from build123d import *

# Parameters (mm, degrees)
F1_DEPTH      = 68.834
F3_DEPTH      = 56.642
F4_DEPTH      = 21.59
F6_DEPTH      = 16.256
F7_T1_DEPTH   = 134.6089194051
F8_SIZE       = 5.08
F9_T4_DEPTH   = 246.1695934192
F9_T9_DEPTH   = 246.1695934192
F11_DEPTH     = 13.97
F12_T1_DEPTH  = 239.1129526059
F12_T6_DEPTH  = 239.1129526059
F13_W         = 8.2417714845
F13_H         = 1.1003240943
F14_DEPTH     = 1.524
F16_DEPTH     = 13.208
F17_T1_DEPTH  = 236.9807138407
F17_T6_DEPTH  = 236.9807138407
F17_T12_DEPTH = 236.9807138407
F17_T18_DEPTH = 236.9807138407


# Not quite as in the source:
# - a fillet or chamfer that OpenCascade refuses, or shapes differently, is made with other operations: its cross-section is extruded or revolved along the edge and cut away or added


with BuildPart() as f1:
    # F0 (on Front) → F1 (new body)
    with BuildSketch(Plane.XZ):
        with BuildLine():
            Line((-134.6334815025, -70.4434812069), (236.5282326937, -70.4434812069))
            Line((236.5282326937, -70.4434812069), (201.5823870897, -52.4187758565))
            add(Edge.make_bspline(
                [(201.5823870897, -52.4187758565), (186.6945113423, -52.7201094998), (157.86128429, -53.3036998994), (136.5029788289, -38.0790520799), (126.1729151011, -30.7155661285)],
                knots=[0, 0, 0, 0, 0.5163444147, 1, 1, 1, 1], degree=3))
            Line((126.1729151011, -30.7155661285), (57.3847740889, -6.4373956993))
            Line((57.3847740889, -6.4373956993), (-104.8375442624, -52.4187758565))
            Line((-104.8375442624, -52.4187758565), (-134.6334815025, -70.4434812069))
        make_face()
    extrude(amount=-F1_DEPTH)

    # F2 (on face) → F3 (join)
    with BuildSketch(Plane(origin=(0, 68.834, 0), x_dir=(-1, 0, 0), z_dir=(0, 1, 0))):
        Polygon((104.8375442624, -52.4187758565), (-57.3847740889, -6.4373956993), (-57.3847740889, -70.4434812069), (134.6334815025, -70.4434812069), align=None)
    extrude(amount=F3_DEPTH)

    # F4 (add): a face of the model
    f4_faces = [f1.faces().sort_by_distance(p)[0] for p in [
        (117.597457412, 68.834, -49.4942566091),
    ]]
    extrude(f4_faces, amount=F4_DEPTH)

    # F5 (on face) → F6 (join)
    with BuildSketch(Plane(origin=(0, 90.424, 0), x_dir=(-1, 0, 0), z_dir=(0, 1, 0))):
        Polygon((-284.8027348518, -56.1655424535), (-284.8027348518, -70.4434812069), (-57.3847740889, -70.4434812069), (-57.3847740889, 0), align=None)
    extrude(amount=F6_DEPTH)

    # F7: chamfer of 22.86 x 14.478 on 1 edges, made by hand

    # F7_s2 → F7_t1 (cut)
    with BuildSketch(Plane.XZ.offset(-165.8564597025)):
        Polygon((262.6095480908, -50.6844785612), (284.8027348518, -70.6435424535), (284.8027348518, -56.1655424535), align=None)
    extrude(amount=F7_T1_DEPTH, mode=Mode.SUBTRACT)

    # F8
    f8_edges = [f1.edges().sort_by_distance(p)[0] for p in [
        (57.384774, 98.552, 0),
    ]]
    chamfer(f8_edges, length=F8_SIZE)

    # F9: fillet of radius 7.971733183 on 2 edges, made by hand


with BuildPart() as f9_tool2:
    # F9_s3 → F9_t4 (new body)
    with BuildSketch(Plane(origin=(39.6696512747, 0, -9.7972362223), x_dir=(0, 1, 0), z_dir=(0.970830567, 0, -0.2397665745))):
        with BuildLine():
            ThreePointArc((106.68, 5.7872175269), (104.3451334085, 11.4240841184), (98.708266817, 13.7589507099))
            Line((98.708266817, 13.7589507099), (106.68, 13.7589507099))
            Line((106.68, 13.7589507099), (106.68, 5.7872175269))
        make_face()
    extrude(amount=F9_T4_DEPTH)

    split(bisect_by=Plane.YZ.offset(57.3847740889), keep=Keep.TOP)


with BuildPart() as f1_1:
    add(f1.part)

    # F9_t1: cut F9_tool2
    add(f9_tool2.part, mode=Mode.SUBTRACT)


with BuildPart() as f9_tool7:
    # F9_s8 → F9_t9 (new body)
    with BuildSketch(Plane(origin=(39.6696512747, 0, -9.7972362223), x_dir=(0, 1, 0), z_dir=(0.970830567, 0, -0.2397665745))):
        with BuildLine():
            ThreePointArc((90.424, 5.7872175269), (92.7588665915, 11.4240841184), (98.395733183, 13.7589507099))
            Line((98.395733183, 13.7589507099), (90.424, 13.7589507099))
            Line((90.424, 13.7589507099), (90.424, 5.7872175269))
        make_face()
    extrude(amount=F9_T9_DEPTH)

    split(bisect_by=Plane(origin=(4.3361166105, 0, 12.285662205), x_dir=(0, 1, 0), z_dir=(0.3328201545, 0, 0.9429903206)), keep=Keep.TOP)


with BuildPart() as f1_2:
    add(f1_1.part)

    # F9_t6: cut F9_tool7
    add(f9_tool7.part, mode=Mode.SUBTRACT)

    # F10 (on face) → F11 (join)
    with BuildSketch(Plane(origin=(0, 125.476, 0), x_dir=(-1, 0, 0), z_dir=(0, 1, 0))):
        Polygon((-45.8267219365, -2.2306151222), (-57.3847740889, -6.4373956993), (104.8375442624, -52.4187758565), (134.6334815025, -70.4434812069), (161.1742377281, -70.4434812069), (150.1698791981, -52.4187758565), align=None)
    extrude(amount=-F11_DEPTH)

    # F12: fillet of radius 7.3585229381 on 2 edges, made by hand

    # F12_s2 → F12_t1 (cut)
    with BuildSketch(Plane(origin=(-171.3471837913, 0, -43.8762710766), x_dir=(0, 1, 0), z_dir=(0.9687439392, 0, 0.2480628554))):
        with BuildLine():
            ThreePointArc((118.1174770619, -13.5288023788), (123.3207385309, -15.6840638479), (125.476, -20.8873253169))
            Line((125.476, -20.8873253169), (125.476, -13.5288023788))
            Line((125.476, -13.5288023788), (118.1174770619, -13.5288023788))
        make_face()
    extrude(amount=F12_T1_DEPTH, mode=Mode.SUBTRACT)


with BuildPart() as f12_tool4:
    # F12_s5 → F12_t6 (new body)
    with BuildSketch(Plane(origin=(-171.3471837913, 0, -43.8762710766), x_dir=(0, 1, 0), z_dir=(0.9687439392, 0, 0.2480628554))):
        with BuildLine():
            ThreePointArc((118.8645229381, -13.5288023788), (113.6612614691, -15.6840638479), (111.506, -20.8873253169))
            Line((111.506, -20.8873253169), (111.506, -13.5288023788))
            Line((111.506, -13.5288023788), (118.8645229381, -13.5288023788))
        make_face()
    extrude(amount=F12_T6_DEPTH)

    split(bisect_by=Plane(origin=(5.9565096776, 0, -21.0145673287), x_dir=(0, 1, 0), z_dir=(-0.272703532, 0, 0.9620981154)), keep=Keep.TOP)


with BuildPart() as f1_3:
    add(f1_2.part)

    # F12_t3: cut F12_tool4
    add(f12_tool4.part, mode=Mode.SUBTRACT)

    # F13 (on face) → F14 (join)
    with BuildSketch(Plane(origin=(5.9565096776, 0, -21.0145673287), x_dir=(0.9620981154, 0, 0.272703532), z_dir=(-0.272703532, 0, 0.9620981154))):
        with Locations((49.3333967155, 86.9543515146)):
            Rectangle(F13_W, F13_H)
    extrude(amount=F14_DEPTH)

    # F15 (on face) → F16 (join)
    with BuildSketch(Plane.XZ.offset(-86.4041894674)):
        Polygon((-104.8238277435, -52.4797327816), (57.3847740889, -6.4373956993), (46.4603118598, -2.0644166507), (-150.4420638084, -52.4797327816), (-161.1757725477, -70.3692361712), (-134.1178864241, -70.3692361712), align=None)
    extrude(amount=F16_DEPTH)

    # F17: fillet of radius 6.7453126933 on 2 edges, made by hand

    # F17_s2 → F17_t1 (cut)
    with BuildSketch(Plane(origin=(59.4421171299, 0, 15.219690044), x_dir=(0, 1, 0), z_dir=(-0.9687495941, 0, -0.2480407708))):
        with BuildLine():
            ThreePointArc((73.1961894674, 20.2692670518), (75.1718458141, 15.4996107052), (79.9415021607, 13.5239543585))
            Line((79.9415021607, 13.5239543585), (73.1961894674, 13.5239543585))
            Line((73.1961894674, 13.5239543585), (73.1961894674, 20.2692670518))
        make_face()
    extrude(amount=F17_T1_DEPTH, mode=Mode.SUBTRACT)


with BuildPart() as f17_tool4:
    # F17_s5 → F17_t6 (new body)
    with BuildSketch(Plane(origin=(59.4421171299, 0, 15.219690044), x_dir=(0, 1, 0), z_dir=(-0.9687495941, 0, -0.2480407708))):
        with BuildLine():
            ThreePointArc((86.4041894674, 20.2692670518), (84.4285331208, 15.4996107052), (79.6588767742, 13.5239543585))
            Line((79.6588767742, 13.5239543585), (86.4041894674, 13.5239543585))
            Line((86.4041894674, 13.5239543585), (86.4041894674, 20.2692670518))
        make_face()
    extrude(amount=F17_T6_DEPTH)

    split(bisect_by=Plane(origin=(43.4988715987, 0, 12.3296114352), x_dir=(0, 1, 0), z_dir=(0.9620981154, 0, 0.272703532)), keep=Keep.TOP)

    split(bisect_by=Plane(origin=(5.5409094947, 0, -19.5483298008), x_dir=(0, 1, 0), z_dir=(-0.272703532, 0, 0.9620981154)), keep=Keep.TOP)


with BuildPart() as f1_4:
    add(f1_3.part)

    # F17_t3: cut F17_tool4
    add(f17_tool4.part, mode=Mode.SUBTRACT)


with BuildPart() as f17_tool10:
    # F17_s11 → F17_t12 (new body)
    with BuildSketch(Plane(origin=(59.4421171299, 0, 15.219690044), x_dir=(0, 1, 0), z_dir=(-0.9687495941, 0, -0.2480407708))):
        with BuildLine():
            ThreePointArc((86.4041894674, 20.2692670518), (84.4285331208, 15.4996107052), (79.6588767742, 13.5239543585))
            Line((79.6588767742, 13.5239543585), (86.4041894674, 13.5239543585))
            Line((86.4041894674, 13.5239543585), (86.4041894674, 20.2692670518))
        make_face()
    extrude(amount=F17_T12_DEPTH)

    split(bisect_by=Plane(origin=(43.4988715987, 0, 12.3296114352), x_dir=(0, 1, 0), z_dir=(-0.9620981154, 0, -0.272703532)), keep=Keep.TOP)

    split(bisect_by=Plane(origin=(5.5409094947, 0, -19.5483298008), x_dir=(0, 1, 0), z_dir=(0.272703532, 0, -0.9620981154)), keep=Keep.TOP)


with BuildPart() as f1_5:
    add(f1_4.part)

    # F17_t9: cut F17_tool10
    add(f17_tool10.part, mode=Mode.SUBTRACT)


with BuildPart() as f17_tool16:
    # F17_s17 → F17_t18 (new body)
    with BuildSketch(Plane(origin=(59.4421171299, 0, 15.219690044), x_dir=(0, 1, 0), z_dir=(-0.9687495941, 0, -0.2480407708))):
        with BuildLine():
            ThreePointArc((86.4041894674, 20.2692670518), (84.4285331208, 15.4996107052), (79.6588767742, 13.5239543585))
            Line((79.6588767742, 13.5239543585), (86.4041894674, 13.5239543585))
            Line((86.4041894674, 13.5239543585), (86.4041894674, 20.2692670518))
        make_face()
    extrude(amount=F17_T18_DEPTH)

    split(bisect_by=Plane(origin=(43.4988715987, 0, 12.3296114352), x_dir=(0, 1, 0), z_dir=(-0.9620981154, 0, -0.272703532)), keep=Keep.TOP)

    split(bisect_by=Plane(origin=(5.5409094947, 0, -19.5483298008), x_dir=(0, 1, 0), z_dir=(-0.272703532, 0, 0.9620981154)), keep=Keep.TOP)


with BuildPart() as f1_6:
    add(f1_5.part)

    # F17_t15: cut F17_tool16
    add(f17_tool16.part, mode=Mode.SUBTRACT)


solid = f1_6.part
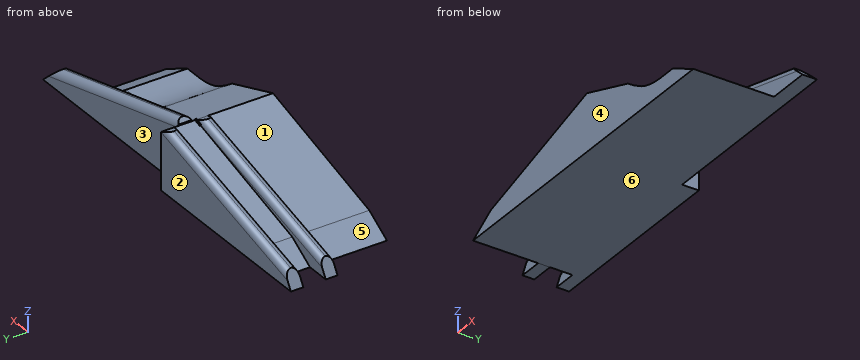
Work out the finished part from the listing and answer in its coordinate system (mm). Face numbers are marked on the shaded views. A direction names the side the tool comes from. Coordinates: 2 decimals unless noted, no trailing zeros. Order: outer loops, then holes, each group sorted by start corner. A loop starts at its lowest first (then second) coordinate and runs counter-clockwise, first axis right, second up. Notation, with made-up numbers: (35.5, 73.25) - (76.5, 73.25) arc R21 ccw to (76.5, 101.25) - close; hole circle Ø6 at (-35, 19.25). An arc over 180 degrees is marked (long way). Put each result on its own line as item: value. Start each with the question number.
1) Flat-ended cylindrical pins translate along their axes: pin 1 (19 mm diameter, centred on x = -79.5, z = -29.5, fed in from -Y); pin 2 (2 mm diameter, centred on x = 128, z = -21.5, fed in from -Y); pin 3 (5.5 mm diameter, centred on y = 114.5, z = -40.5, fed in from +X). Find the tip coordinate at first contact, or state that the pin passes through.
2) Find section A-A (z = -66). Give the vertices of the cut face in (x, y).
3) For a pull along Y with two mould halves and no side action, classify the marked faces 3, 4, 5 and 6 as released by +Y, released by -Y, zero draft, split by the parting line, or undercut.
4) For the marked faces 1 and 2, determine the directions among +Z, -Z, +X, -X, +Y, -Y from which every point of the face is accessible in a straight line to the end or side of a thin tool.
5) Find the intervals of material crossed by line 1 (Y direction, x = -1.5, z = -22); line 2 (Y direction, x = 162, z = -60); line 3 (Z direction, x = 201, y = 25.5), in increasing order. Write a range as from..to.
Results list:
1. pin 1: stops at y = 73.47
1. pin 2: stops at y = 91.02
1. pin 3: stops at x = 57.38
2. outline: (-158.55, 73.2) - (-127.29, 73.2) - (-127.29, 0) - (227.91, 0) - (227.91, 90.42) - (279.64, 90.42) - (279.64, 106.68) - (57.38, 106.68) - (57.38, 125.48) - (-158.46, 125.48) - (-158.46, 111.51) - (-127.29, 111.51) - (-127.29, 86.4) - (-158.55, 86.4) - close
3. face 3: released by +Y
3. face 4: released by -Y
3. face 5: undercut
3. face 6: zero draft
4. face 1: +Z, -X, -Y
4. face 2: +Z, -Z, +X, -X, +Y
5. line 1: y = 73.2..86.4, 111.51..125.48
5. line 2: y = 0..106.68
5. line 3: z = -70.44..-52.43
